Geometry: final body of the model. Coordinates: model frame, mm. Face numbers are marked on the shaded views. A direction names the side the tool comes from. Coordinates: 2 decimals unless noted, no trailing zeros. Loops run counter-clockwise (first coordinate to the right, second up) from the corner with the lowest first, then second, coordinate; pieces in that order, holes last. Notation, with made-up numbers: (56.25, -0.5) - (113.25, -0.5) arc R17 cw to (113.25, 22.5) - close; hole circle Ø4 at (-10.5, -20.5). An arc over 180 degrees is marked (long way). Write each question's results on one line, items separated by ' | '. Start each with the question number.
from build123d import *

# Parameters (mm, degrees)
SKETCH1_R           = 22.5
BOSS_EXTRUDE1_DEPTH = 15
SKETCH2_R           = 6.75
CUT_EXTRUDE1_DEPTH  = 10
SKETCH3_R           = 2
CUT_EXTRUDE2_DEPTH  = 35
CIRPATTERN1_COUNT   = 4
SKETCH6_R           = 1.75
CUT_EXTRUDE4_DEPTH  = 45
BOSS_EXTRUDE2_START = 6
SKETCH7_R           = 5
SKETCH7_R_2         = 1.75
BOSS_EXTRUDE2_DEPTH = 6
FILLET1_R           = 1
SKETCH8_R           = 3.5
CUT_EXTRUDE5_DEPTH  = 5


with BuildPart() as part:
    # Sketch1 → Boss-Extrude1 (new body)
    with BuildSketch(Plane(origin=(0, 0, 0), x_dir=(1, 0, 0), z_dir=(0, 1, 0))):
        with Locations(Location((0, 0, 0), (0, 0, 270))):
            Circle(SKETCH1_R)
    extrude(amount=BOSS_EXTRUDE1_DEPTH)

    # Sketch2 → Cut-Extrude1 (cut)
    with BuildSketch(Plane(origin=(0, 15, 0), x_dir=(1, 0, 0), z_dir=(0, 1, 0))):
        with Locations(Location((0, 13, 0), (0, 0, 270))):
            Circle(SKETCH2_R)
    cut_extrude1 = extrude(amount=-CUT_EXTRUDE1_DEPTH, mode=Mode.SUBTRACT)

    # Sketch3 → Cut-Extrude2 (cut)
    with BuildSketch(Plane(origin=(0, 5, 0), x_dir=(1, 0, 0), z_dir=(0, 1, 0))):
        with Locations(Location((0, 13, 0), (0, 0, 270))):
            Circle(SKETCH3_R)
    cut_extrude2 = extrude(amount=-CUT_EXTRUDE2_DEPTH, mode=Mode.SUBTRACT)

    # CirPattern1: Cut-Extrude1, Cut-Extrude2 ×4 about axis
    cirpattern1_axis = Axis((0, 0, 0), (0, 1, 0))
    add([cut_extrude1.rotate(cirpattern1_axis, i * 360 / CIRPATTERN1_COUNT) for i in range(1, CIRPATTERN1_COUNT)], mode=Mode.SUBTRACT)
    add([cut_extrude2.rotate(cirpattern1_axis, i * 360 / CIRPATTERN1_COUNT) for i in range(1, CIRPATTERN1_COUNT)], mode=Mode.SUBTRACT)

    # Sketch6 → Cut-Extrude4 (cut)
    with BuildSketch(Plane(origin=(0, 15, 0), x_dir=(1, 0, 0), z_dir=(0, 1, 0))):
        with Locations(Location((0, 0, 0), (0, 0, 270))):
            Circle(SKETCH6_R)
    extrude(amount=-CUT_EXTRUDE4_DEPTH, mode=Mode.SUBTRACT)

    # Sketch7 → Boss-Extrude2 (add)
    with BuildSketch(Plane(origin=(0, 15, 0), x_dir=(1, 0, 0), z_dir=(0, 1, 0)).offset(BOSS_EXTRUDE2_START)):
        with Locations(Location((0, 0, 0), (0, 0, 270))):
            Circle(SKETCH7_R)
        with Locations(Location((0, 0, 0), (0, 0, 270))):
            Circle(SKETCH7_R_2, mode=Mode.SUBTRACT)
    extrude(amount=-BOSS_EXTRUDE2_DEPTH)

    # Fillet1
    fillet1_edges = [part.edges().sort_by_distance(p)[0] for p in [
        (0, 15, -5),
    ]]
    fillet(fillet1_edges, radius=FILLET1_R)

    # Sketch8 → Cut-Extrude5 (cut)
    with BuildSketch(Plane.XZ):
        with Locations(Location((0, 0, 0), (0, 0, 270))):
            Circle(SKETCH8_R)
    extrude(amount=-CUT_EXTRUDE5_DEPTH, mode=Mode.SUBTRACT)


solid = part.part
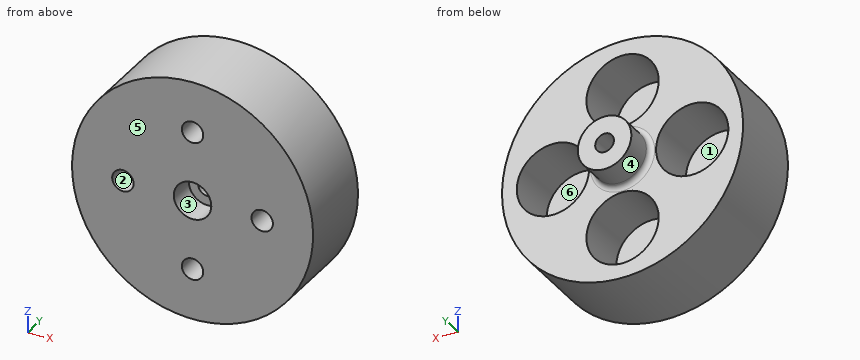
1) Material intervals for line 1 (Z direction, x = 1.5, y = 10.75); line 2 (Y direction, x = -9, z = 10); line 3 (X direction, y = 8, z = 4), sorted ascending. Write a range as [from, to].
2) Pin query (flat end, axial travel): pin 1 Ø5 at (x, y) = (-13, 13) entering from -Z; pin 2 Ø6 at (y, z) = (18.5, -0.5) entering from -X; pin 3 Ø1.5 at (x, y) = (-13.5, 8.5) entering from -Z. Return the tip coordinate at first contact, or that it passes through.
3) Access query for the marked faces 1, 2 and 3. Directions: +Z, -Z, +X, -X, +Y, -Y. A direction counts if a zero-diameter tool reaches every point of the face in a straight line with its end or side. Return the directions, or none.
4) Section query C-C on x = -13. Output: boundary loops of the cut face in (y, z), and give its area (3 significant figures).
5) Section query D-D on z = -12. Output: boundary loops of the cut face in (x, y).
6) Section query A-A on x = 0. Count the separate pieces of the cut face and the enclosed holes in it, and give its area (3 significant figures).
7) Pull-direction query (X, two-part tool) for the marked faces 4, 5 and 6; classes: released by +X, released by -X, zero draft, split by the parting line, or undercut.
Returned:
1) line 1: z = [-22.45, -19.58], [-6.42, -0.9], [0.9, 6.42], [19.58, 22.45] | line 2: y = [0, 15] | line 3: x = [-22.14, -18.44], [-7.56, 7.56], [18.44, 22.14]
2) pin 1: stops at z = -19.9 | pin 2: stops at x = -5.12 | pin 3: stops at z = -18.54
3) face 1: +Y | face 2: +Y, -Y | face 3: -Y
4) outline: (0, -18.36) - (15, -18.36) - (15, -6.75) - (5, -6.75) - (5, -2) - (0, -2) - close; (0, 2) - (5, 2) - (5, 6.75) - (15, 6.75) - (15, 18.36) - (0, 18.36) - close | area: 396 mm²
5) outline: (-19.03, 0) - (-1.73, 0) - (-1.73, 5) - (-6.68, 5) - (-6.68, 15) - (-19.03, 15) - close; (1.73, 0) - (19.03, 0) - (19.03, 15) - (6.68, 15) - (6.68, 5) - (1.73, 5) - close
6) separate pieces: 4 | enclosed holes: 0 | area: 334 mm²
7) face 4: split by the parting line | face 5: zero draft | face 6: undercut
